Build history of the part. All positions in model axes, mm. A direction names the side the tool comes from. Round coordinates to 2 decimals unless told otherwise and drop trailing zeros. Loops run counter-clockwise (first coordinate to the right, second up) from the corner with the lowest first, then second, coordinate; pieces in that order, holes last. Notation, with made-up numbers: (6, 8) - (42, 8) arc R19 ccw to (42, 23) - close; hole circle Ø10 at (74, 52). An arc over 180 degrees is marked (long way). One line per question, with ' | ' between items. Start each with the question number.
from build123d import *

# Parameters (mm, degrees)
SKETCH_1_W      = 28
SKETCH_1_H      = 28
SKETCH_1_R      = 1.25
EXTRUDE_1_DEPTH = 41
SKETCH_2_R      = 11
EXTRUDE_2_DEPTH = 3
SKETCH_3_R      = 2.5
EXTRUDE_3_DEPTH = 20
FILLET_1_R      = 2


with BuildPart() as part:
    # 草图1 → 凸台-拉伸1 (new body)
    with BuildSketch(Plane.XY):
        Rectangle(SKETCH_1_W, SKETCH_1_H)
        with Locations((-11.5, 11.5)):
            Circle(SKETCH_1_R, mode=Mode.SUBTRACT)
        with Locations((11.5, 11.5)):
            Circle(SKETCH_1_R, mode=Mode.SUBTRACT)
        with Locations((11.5, -11.5)):
            Circle(SKETCH_1_R, mode=Mode.SUBTRACT)
        with Locations((-11.5, -11.5)):
            Circle(SKETCH_1_R, mode=Mode.SUBTRACT)
    extrude(amount=EXTRUDE_1_DEPTH)

    # 草图2 → 凸台-拉伸2 (add)
    with BuildSketch(Plane.XY.offset(41)):
        Circle(SKETCH_2_R)
    extrude(amount=EXTRUDE_2_DEPTH)

    # 草图3 → 凸台-拉伸3 (add)
    with BuildSketch(Plane.XY.offset(44)):
        Circle(SKETCH_3_R)
    extrude(amount=EXTRUDE_3_DEPTH)

    # 圆角1
    fillet_1_edges = [part.edges().sort_by_distance(p)[0] for p in [
        (14, -14, 20.5),
        (-14, -14, 20.5),
        (-14, 14, 20.5),
        (14, 14, 20.5),
    ]]
    fillet(fillet_1_edges, radius=FILLET_1_R)


solid = part.part
1) Drop flat-ended pins along their axis: pin 1 (3 mm diameter, centred on x = -11.5, y = -11.5, fed in from +Z); pin 2 (1 mm diameter, centred on y = -0.5, z = 43.5, fed in from +X). Give the stop position or say it passes through.
2) Saw through at B-B on y = 0. Write the cut outline in (x, z), and give its area (3 significant figures).
3) Saw through at A-A on z = 16.5. Write the cut outline in (x, y), and give its area (3 significant figures).
4) Saw through at D-D on z = 60. Write the cut outline in (x, y), and give its area (3 significant figures).
5) Two-plate mould, pull along Y, no slides. Class faces 3 (the cylindrical face through (-12.421, 12.345, 20.213)), 4 (the flat face through (-6, 10, 41)), 5 (the cylindrical face through (-2.38, -10.74, 42.48)), 6 (the flat face through (0, 14, 20)): +Y half, -Y half, draft (parallel to the pull), parting line (faces both ways), or undercut.
6) Wall check: line 1 (Y direction, x = 12, z = 36); line 2 (Y direction, x = -12.5, z = 9); line 3 (Z direction, x = -9, y = 6). Give the ranges that are in metal, low to high. Write a range as [from, to].
7) Tool access for faces 1 (the cylindrical face through (-13.43, -13.4, 20.79)), 2 (the cylindrical face through (-0.54, -2.44, 53.86)): list every direction of +Z, -Z, +X, -X, +Y, -Y with a clear straight run to the whole face (end or side of a thin tool).
Answer key:
1) pin 1: z = 41 | pin 2: x = 11
2) outline: (-14, 0) - (14, 0) - (14, 41) - (11, 41) - (11, 44) - (2.5, 44) - (2.5, 64) - (-2.5, 64) - (-2.5, 44) - (-11, 44) - (-11, 41) - (-14, 41) - close | area: 1,310 mm²
3) outline: (-14, -12) arc R2 ccw to (-12, -14) - (12, -14) arc R2 ccw to (14, -12) - (14, 12) arc R2 ccw to (12, 14) - (-12, 14) arc R2 ccw to (-14, 12) - close; hole circle Ø2.5 at (-11.5, -11.5); hole circle Ø2.5 at (-11.5, 11.5); hole circle Ø2.5 at (11.5, -11.5); hole circle Ø2.5 at (11.5, 11.5) | area: 761 mm²
4) outline: circle Ø5 at (0, 0) | area: 19.6 mm²
5) face 3: undercut | face 4: draft | face 5: parting line | face 6: +Y half
6) line 1: [-14, -12.65], [-10.35, 10.35], [12.65, 14] | line 2: [-13.94, -12.25], [-10.75, 10.75], [12.25, 13.94] | line 3: [0, 44]
7) face 1: +Z, -Z, -X, -Y | face 2: +Z
